```python
from build123d import *

# Parameters (mm, degrees)
F0_W     = 25.4
F0_H     = 63.5
F1_DEPTH = 5.588
F2_R     = 5.08
F3_R     = 12.7
F4_R     = 5.08
F5_R     = 19.04999


# Not quite as in the source:
# - a fillet or chamfer is up to 0.001 mm smaller than in the source, because OpenCascade refuses the exact size


with BuildPart() as f1:
    # F0 (on Top) → F1 (new body)
    with BuildSketch(Plane.XY):
        Polygon((38.1, 12.7), (-38.1, 12.7), (-38.1, -12.7), (-12.7, -12.7), (12.7, -12.7), (38.1, -12.7), align=None)
        with Locations((0, -44.45)):
            Rectangle(F0_W, F0_H)
        Polygon((12.7, -76.2), (-12.7, -76.2), (-19.05, -76.2), (-19.05, -114.3), (19.05, -114.3), (19.05, -76.2), align=None)
    extrude(amount=F1_DEPTH)

    # F2
    f2_edges = [f1.edges().sort_by_distance(p)[0] for p in [
        (-38.1, -12.7, 2.794),
        (38.1, -12.7, 2.794),
    ]]
    fillet(f2_edges, radius=F2_R)

    # F3
    f3_edges = [f1.edges().sort_by_distance(p)[0] for p in [
        (-12.7, -12.7, 2.794),
        (12.7, -12.7, 2.794),
    ]]
    fillet(f3_edges, radius=F3_R)

    # F4
    f4_edges = [f1.edges().sort_by_distance(p)[0] for p in [
        (-12.7, -76.2, 2.794),
        (12.7, -76.2, 2.794),
    ]]
    fillet(f4_edges, radius=F4_R)

    # F5 (radius 19.05 in the source; OpenCascade refuses exactly that, so slightly less here)
    f5_edges = [f1.edges().sort_by_distance(p)[0] for p in [
        (-19.05, -114.3, 2.794),
        (-19.05, -76.2, 2.794),
        (19.05, -114.3, 2.794),
        (19.05, -76.2, 2.794),
    ]]
    fillet(f5_edges, radius=F5_R)


solid = f1.part
```
Part model, mm, in its own coordinate system. A direction names the side the tool comes from. Give positions to 0.01 mm unless a question says otherwise; leave off trailing zeros. Order: outer loops, then holes, each group sorted by start corner. A loop starts at its lowest first (then second) coordinate and runs counter-clockwise, first axis right, second up. Notation, with made-up numbers: M -12.5,57 L -4.5,57 A24 cw -4.5,76 Z; hole C -27,52.5 d6. An arc over 180 degrees is marked long. Use a Markdown table: item, result. Add a question column.
(1) Probe line 1 along Y through (x, z) = (-28, 3.7); line 2 along X through (y, z) = (-87.5, 3.9). List the from-to ranges inside material, lowest first. Write a range as [from, to].
(2) Mould opens along Y. For faces 6 (the face through (-36.651, -11.172, 2.833)), 7 (the face through (-13.036, -72.938, 2.833)), 8 (the face through (-38.1, 3, 3)) say: +Y half, -Y half, draft (parallel to the pull), parting line (faces both ways), or undercut.
(3) Saw through at A-A, the plane x = 31. Give the cut face in (y, z), and give its area (3 significant figures).
(4) 3-axis set-ups, long thin cutter, end or side, ignore diameter. For faces 1 (the face through (1, 12.7, 3)), 2 (the face through (19.05, -91, 3)), 3 (the face through (16.52, -16.32, 2.83)), 4 (the face through (-19.05, -91, 3)), 5 (the face through (-12.7, -49, 3)): which of +Z, -Z, +X, -X, +Y, -Y reach the whole face in a straight line?
(5) Drop flat-ended pins along their axis: P1, Ø3, axis at y = -41.5, z = 1.5, coming from the +X side; P2, Ø1.7, axis at y = -93, z = 3, coming from the -X side; P3, Ø1, axis at y = -72, z = 3.5, coming from the -X side. Give the stop position or say it passes through.
Answer key:
| question | item | result |
|---|---|---|
| 1 | line 1 | [-12.7, 12.7] |
| 1 | line 2 | [-19.05, 19.05] |
| 2 | face 6 | -Y half |
| 2 | face 7 | undercut |
| 2 | face 8 | draft |
| 3 | outline | M -12.7,0 L 12.7,0 L 12.7,5.59 L -12.7,5.59 Z |
| 3 | area | 142 mm^2 |
| 4 | face 1 | +Z, -Z, +X, -X, +Y |
| 4 | face 2 | +Z, -Z, +X, -Y |
| 4 | face 3 | +Z, -Z, +X |
| 4 | face 4 | +Z, -Z, -X, -Y |
| 4 | face 5 | +Z, -Z, -X |
| 5 | P1 | x = 12.7 |
| 5 | P2 | x = -19.05 |
| 5 | P3 | x = -12.89 |
